```python
from build123d import *

# Parameters (mm, degrees)
SKETCH1_R           = 72.5
BOSS_EXTRUDE1_DEPTH = 19
SKETCH2_R           = 20
CUT_EXTRUDE1_DEPTH  = 105.276075876
SKETCH3_R           = 6.517224347
CUT_EXTRUDE2_DEPTH  = 15.276014
CIRPATTERN1_START   = 3.72398555
CIRPATTERN1_DEPTH   = 15.27601445


# Read off the part's stored shape, not the designer's step: CirPattern1
with BuildPart() as part:
    # Sketch1 → Boss-Extrude1 (new body)
    with BuildSketch(Plane(origin=(0, 0, 0), x_dir=(1, 0, 0), z_dir=(0, 1, 0))):
        with Locations(Location((0, 0, 0), (0, 0, 270))):
            Circle(SKETCH1_R)
    extrude(amount=BOSS_EXTRUDE1_DEPTH)

    # Sketch2 → Cut-Extrude1 (cut, through all)
    with BuildSketch(Plane(origin=(0, 0, 0), x_dir=(1, 0, 0), z_dir=(0, 1, 0))):
        with Locations(Location((0, 0, 0), (0, 0, 270))):
            Circle(SKETCH2_R)
    extrude(amount=CUT_EXTRUDE1_DEPTH, mode=Mode.SUBTRACT)

    # Sketch3 → Cut-Extrude2 (cut)
    with BuildSketch(Plane(origin=(0, 19, 0), x_dir=(1, 0, 0), z_dir=(0, 1, 0))):
        with Locations((-18.137210473, 0)):
            Circle(SKETCH3_R)
    extrude(amount=-CUT_EXTRUDE2_DEPTH, mode=Mode.SUBTRACT)

    # CirPattern1 outline → CirPattern1 (cut)
    with BuildSketch(Plane(origin=(0, 0, 0), x_dir=(1, 0, 0), z_dir=(0, 1, 0)).offset(CIRPATTERN1_START)):
        with BuildLine():
            ThreePointArc((-3.859650179, -19.624043938), (-10, -17.320508076), (-15.065095486, -13.154577074))
            ThreePointArc((-15.065095486, -13.154577074), (-12.32721741, -21.35136687), (-3.859650179, -19.624043938))
        make_face()
        with BuildLine():
            ThreePointArc((-3.859650179, 19.624043938), (-12.32721741, 21.35136687), (-15.065095486, 13.154577074))
            ThreePointArc((-15.065095486, 13.154577074), (-10, 17.320508076), (-3.859650179, 19.624043938))
        make_face()
        with BuildLine():
            ThreePointArc((15.065095486, -13.154577074), (10, -17.320508076), (3.859650179, -19.624043938))
            ThreePointArc((3.859650179, -19.624043938), (12.32721741, -21.35136687), (15.065095486, -13.154577074))
        make_face()
        with BuildLine():
            ThreePointArc((15.065095486, 13.154577074), (12.32721741, 21.35136687), (3.859650179, 19.624043938))
            ThreePointArc((3.859650179, 19.624043938), (10, 17.320508076), (15.065095486, 13.154577074))
        make_face()
        with BuildLine():
            ThreePointArc((18.924745665, 6.469466864), (20, 0), (18.924745665, -6.469466864))
            ThreePointArc((18.924745665, -6.469466864), (24.65443482, 0), (18.924745665, 6.469466864))
        make_face()
    extrude(amount=CIRPATTERN1_DEPTH, mode=Mode.SUBTRACT)


solid = part.part
```
Part model, mm, in its own coordinate system. A direction names the side the tool comes from. Round coordinates to 2 decimals unless told otherwise and drop trailing zeros. Order: outer loops, then holes, each group sorted by start corner. A loop starts at its lowest first (then second) coordinate and runs counter-clockwise, first axis right, second up. Notation, with made-up numbers: M 41,-23.75 L 97,-23.75 A21 ccw 97,-19.75 Z; hole C 56,15 d1. An arc over 180 degrees is marked long. Put each result on its own line as item: value. Start each with the question number.
1. Slice it at A-A on z = 0. List the corners of the cut face in (x, y), then the cut area to 3 significant figures.
2. Slice it at D-D on z = -24.5. List the corners of the cut face in (x, y), then the cut area to 3 significant figures.
3. Drill centre lines: probe 1 along X at (y, z) = (14.5, 0); probe 2 along Y at (x, z) = (22.5, 1.5); probe 3 along X at (y, z) = (11, -19). Where is each one in solid material? Low to high. Write a range as [from, to].
4. Tool access for faces 4 (the face through (-15, 0, 15)), 5 (the face through (-11, 3.724, -19)): list every direction of +Z, -Z, +X, -X, +Y, -Y with a clear straight run to the whole face (end or side of a thin tool).
5. Two-plate mould, pull along X, no slides. Class faces 1 (the face through (17, 19, 15)), 2 (the face through (21.78, 9.37, 69.15)), 3 (the face through (-24.653, 11.469, -0.132)): +X half, -X half, draft (parallel to the pull), parting line (faces both ways), or undercut.
6. Slice it at B-B on x = 0. List the corners of the cut face in (y, z).
7. Slice it at C-C on y = 14.75. List the corners of the cut face in (x, z).
8. Drop flat-ended pins along their axis: pin 1 (2 mm diameter, centred on x = 2.5, y = 4.5, fed in from -Z); pin 2 (6 mm diameter, centred on x = -30.5, y = 16.5, fed in from +Z); pin 3 (4 mm diameter, centred on x = -50.5, y = 8, fed in from -Z). Give the stop position or say it passes through.
Findings:
1. outline: M -72.5,0 L -20,0 L -20,3.72 L -24.65,3.72 L -24.65,19 L -72.5,19 Z; M 20,0 L 72.5,0 L 72.5,19 L 24.65,19 L 24.65,3.72 L 20,3.72 Z
1. area: 1,850 mm2
2. outline: M -68.23,0 L 68.23,0 L 68.23,19 L -68.23,19 Z
2. area: 2,590 mm2
3. probe 1: [-72.5, -24.65], [24.65, 72.5]
3. probe 2: [0, 3.72]
3. probe 3: [-69.97, -14.69], [14.69, 69.97]
4. face 4: +Z, -Z, +X, -X, -Y
4. face 5: +Y
5. face 1: draft
5. face 2: parting line
5. face 3: undercut
6. outline: M 0,-72.5 L 19,-72.5 L 19,-20 L 0,-20 Z; M 0,20 L 19,20 L 19,72.5 L 0,72.5 Z
7. outline: C 0,0 d145; hole M -18.92,-6.47 A20 ccw -15.07,-13.15 A6.52 ccw -3.86,-19.62 A20 ccw 3.86,-19.62 A6.52 ccw 15.07,-13.15 A20 ccw 18.92,-6.47 A6.52 ccw 18.92,6.47 A20 ccw 15.07,13.15 A6.52 ccw 3.86,19.62 A20 ccw -3.86,19.62 A6.52 ccw -15.07,13.15 A20 ccw -18.92,6.47 A6.52 ccw Z
8. pin 1: z = -72.48
8. pin 2: z = 67.08
8. pin 3: z = -53.89
